Model file for the job. Use its own axes, mm. A direction names the side the tool comes from. Round coordinates to 2 decimals unless told otherwise and drop trailing zeros. Order: outer loops, then holes, each group sorted by start corner. A loop starts at its lowest first (then second) coordinate and runs counter-clockwise, first axis right, second up. Notation, with made-up numbers: M 62.25,80 L 112.25,80 A28 cw 112.25,117 Z; hole C 13,56 d4. An arc over 180 degrees is marked long. Return JSON: item names as keys, results as strings. Group by question number.
Item 1: Pull direction Z, two halves, no side cores. Call faces 1 (the face through (11.745, -3.54, -1.565)), 2 (the face through (0, 2.674, 2)), 3 (the face through (3, 1, 6.975)): pulls with the +Z half, pulls with the -Z half, needs draft (parallel to the pull), parting line crosses it, or undercut.
Item 2: Slice it at D-D on x = 0. Write the cut outline in (y, z) (3 decimals), then the cut area to 3 significant figures.
Item 3: Probe line 1 along Z through (x, y) = (8.25, 1.25) (3 decimals); line 2 along Y through (x, z) = (0, -0.5) (3 decimals); line 3 along Y through (x, z) = (0, 2.75). List the from-to ranges inside material, lowest first.
Item 4: Slice it at A-A on x = 9. Write the cut outline in (y, z) (3 decimals).
Item 5: Slice it at B-B on y = 0. Write the cut outline in (x, z) (1 decimal), then the cut area to 3 significant figures.
Item 6: Pin check, flat tips, straight feed: pin 1 Ø1.1 at (x, z) = (0.5, 1.5) entering from -Y; pin 2 Ø1.1 at (y, z) = (0, 1.5) entering from -X; pin 3 Ø1.9 at (x, z) = (-1, 2.5) entering from +Y. Stop position of each tip, or through.
Item 7: Slice it at C-C on z = -1. Write the cut outline in (x, y) (3 decimals).
Item 8: Which spindle directions (+Z, -Z, +X, -X, +Y, -Y) get a long thin tool onto all of the face, cutting with end or side? Do faces 4 (the face through (0, -2.674, 2)), 5 (the face through (-5.398, 0, 2)), 6 (the face through (-11.795, -3.49, -1.565)). Say none if no direction does.
from build123d import *

# Parameters (mm, degrees)
F0_R      = 1.5
F1_DEPTH  = 3.8
F1_FACE_R = 1.5
F2_DEPTH  = 3.175
F3_R      = 1.5
F4_DEPTH  = 3.175
F5_R      = 1.27
F6_R      = 1.27


with BuildPart() as f1:
    # F0 (on Top) → F1 (new body)
    with BuildSketch(Plane.XY):
        with BuildLine():
            ThreePointArc((5.3975, 2.0388861202), (5.2115128061, 2.4878989263), (4.7625, 2.6738861202))
            Line((4.7625, 2.6738861202), (-4.7625, 2.6738861202))
            ThreePointArc((-4.7625, 2.6738861202), (-5.2115128061, 2.4878989263), (-5.3975, 2.0388861202))
            Line((-5.3975, 2.0388861202), (-5.3975, -2.0388861202))
            ThreePointArc((-5.3975, -2.0388861202), (-5.2115128061, -2.4878989263), (-4.7625, -2.6738861202))
            Line((-4.7625, -2.6738861202), (4.7625, -2.6738861202))
            ThreePointArc((4.7625, -2.6738861202), (5.2115128061, -2.4878989263), (5.3975, -2.0388861202))
            Line((5.3975, -2.0388861202), (5.3975, 2.0388861202))
        make_face()
        Circle(F0_R, mode=Mode.SUBTRACT)
    extrude(amount=F1_DEPTH)

    # F0 (on Top) + F1_face (on face) → F2 (join)
    with BuildSketch(Plane.XY):
        with BuildLine():
            ThreePointArc((12.7, 1.27), (11.7700640303, 3.5150640303), (9.525, 4.445))
            Line((9.525, 4.445), (-9.525, 4.445))
            ThreePointArc((-9.525, 4.445), (-11.7700640303, 3.5150640303), (-12.7, 1.27))
            Line((-12.7, 1.27), (-12.7, -1.27))
            ThreePointArc((-12.7, -1.27), (-11.7700640303, -3.5150640303), (-9.525, -4.445))
            Line((-9.525, -4.445), (9.525, -4.445))
            ThreePointArc((9.525, -4.445), (11.7700640303, -3.5150640303), (12.7, -1.27))
            Line((12.7, -1.27), (12.7, 1.27))
        make_face()
        with BuildLine():
            Line((-4.7625, 2.6738861202), (4.7625, 2.6738861202))
            ThreePointArc((4.7625, 2.6738861202), (5.2115128061, 2.4878989263), (5.3975, 2.0388861202))
            Line((5.3975, 2.0388861202), (5.3975, -2.0388861202))
            ThreePointArc((5.3975, -2.0388861202), (5.2115128061, -2.4878989263), (4.7625, -2.6738861202))
            Line((4.7625, -2.6738861202), (-4.7625, -2.6738861202))
            ThreePointArc((-4.7625, -2.6738861202), (-5.2115128061, -2.4878989263), (-5.3975, -2.0388861202))
            Line((-5.3975, -2.0388861202), (-5.3975, 2.0388861202))
            ThreePointArc((-5.3975, 2.0388861202), (-5.2115128061, 2.4878989263), (-4.7625, 2.6738861202))
        make_face(mode=Mode.SUBTRACT)
    with BuildSketch(Plane(origin=(0, 0, 0), x_dir=(1, 0, 0), z_dir=(0, 0, -1))):
        with BuildLine():
            ThreePointArc((4.7625, -2.6738861202), (5.2115128061, -2.4878989263), (5.3975, -2.0388861202))
            Line((5.3975, -2.0388861202), (5.3975, 2.0388861202))
            ThreePointArc((5.3975, 2.0388861202), (5.2115128061, 2.4878989263), (4.7625, 2.6738861202))
            Line((4.7625, 2.6738861202), (-4.7625, 2.6738861202))
            ThreePointArc((-4.7625, 2.6738861202), (-5.2115128061, 2.4878989263), (-5.3975, 2.0388861202))
            Line((-5.3975, 2.0388861202), (-5.3975, -2.0388861202))
            ThreePointArc((-5.3975, -2.0388861202), (-5.2115128061, -2.4878989263), (-4.7625, -2.6738861202))
            Line((-4.7625, -2.6738861202), (4.7625, -2.6738861202))
        make_face()
        Circle(F1_FACE_R, mode=Mode.SUBTRACT)
    extrude(amount=-F2_DEPTH, dir=(0, 0, 1))

    # F3 (on face) → F4 (join)
    with BuildSketch(Plane.XY.offset(3.8)):
        with BuildLine():
            ThreePointArc((12.7, 1.27), (11.7700640303, 3.5150640303), (9.525, 4.445))
            Line((9.525, 4.445), (-9.525, 4.445))
            ThreePointArc((-9.525, 4.445), (-11.7700640303, 3.5150640303), (-12.7, 1.27))
            Line((-12.7, 1.27), (-12.7, -1.27))
            ThreePointArc((-12.7, -1.27), (-11.7700640303, -3.5150640303), (-9.525, -4.445))
            Line((-9.525, -4.445), (9.525, -4.445))
            ThreePointArc((9.525, -4.445), (11.7700640303, -3.5150640303), (12.7, -1.27))
            Line((12.7, -1.27), (12.7, 1.27))
        make_face()
        with BuildLine():
            ThreePointArc((4.7625, 2.6738861202), (5.2115128061, 2.4878989263), (5.3975, 2.0388861202))
            Line((5.3975, 2.0388861202), (5.3975, -2.0388861202))
            ThreePointArc((5.3975, -2.0388861202), (5.2115128061, -2.4878989263), (4.7625, -2.6738861202))
            Line((4.7625, -2.6738861202), (-4.7625, -2.6738861202))
            ThreePointArc((-4.7625, -2.6738861202), (-5.2115128061, -2.4878989263), (-5.3975, -2.0388861202))
            Line((-5.3975, -2.0388861202), (-5.3975, 2.0388861202))
            ThreePointArc((-5.3975, 2.0388861202), (-5.2115128061, 2.4878989263), (-4.7625, 2.6738861202))
            Line((-4.7625, 2.6738861202), (4.7625, 2.6738861202))
        make_face(mode=Mode.SUBTRACT)
        with BuildLine():
            Line((5.3975, -2.0388861202), (5.3975, 2.0388861202))
            ThreePointArc((5.3975, 2.0388861202), (5.2115128061, 2.4878989263), (4.7625, 2.6738861202))
            Line((4.7625, 2.6738861202), (-4.7625, 2.6738861202))
            ThreePointArc((-4.7625, 2.6738861202), (-5.2115128061, 2.4878989263), (-5.3975, 2.0388861202))
            Line((-5.3975, 2.0388861202), (-5.3975, -2.0388861202))
            ThreePointArc((-5.3975, -2.0388861202), (-5.2115128061, -2.4878989263), (-4.7625, -2.6738861202))
            Line((-4.7625, -2.6738861202), (4.7625, -2.6738861202))
            ThreePointArc((4.7625, -2.6738861202), (5.2115128061, -2.4878989263), (5.3975, -2.0388861202))
        make_face()
        Circle(F3_R, mode=Mode.SUBTRACT)
    extrude(amount=F4_DEPTH)

    # F5
    f5_edges = [f1.edges().sort_by_distance(p)[0] for p in [
        (-1.5, 0, 6.975),
    ]]
    fillet(f5_edges, radius=F5_R)

    # F6
    f6_edges = [f1.edges().sort_by_distance(p)[0] for p in [
        (-1.5, 0, -3.175),
    ]]
    fillet(f6_edges, radius=F6_R)


solid = f1.part
Output values:
{
 "1": {"face 1": "needs draft", "face 2": "undercut", "face 3": "pulls with the +Z half"},
 "2": {"outline": "M -4.445,-3.175 L -2.77,-3.175 A1.27 ccw -1.5,-1.905 L -1.5,5.705 A1.27 ccw -2.77,6.975 L -4.445,6.975 L -4.445,3.8 L -2.674,3.8 L -2.674,0 L -4.445,0 Z; M 1.5,-1.905 A1.27 ccw 2.77,-3.175 L 4.445,-3.175 L 4.445,0 L 2.674,0 L 2.674,3.8 L 4.445,3.8 L 4.445,6.975 L 2.77,6.975 A1.27 ccw 1.5,5.705 Z", "area": "44.9 mm²"},
 "3": {"line 1": "-3.175 to 0, 3.8 to 6.975", "line 2": "-4.445 to -1.5, 1.5 to 4.445", "line 3": "-2.67 to -1.5, 1.5 to 2.67"},
 "4": {"outline": "M -4.445,-3.175 L 4.445,-3.175 L 4.445,0 L -4.445,0 Z; M -4.445,3.8 L 4.445,3.8 L 4.445,6.975 L -4.445,6.975 Z"},
 "5": {"outline": "M -12.7,-3.2 L -2.8,-3.2 A1.3 ccw -1.5,-1.9 L -1.5,5.7 A1.3 ccw -2.8,7 L -12.7,7 L -12.7,3.8 L -5.4,3.8 L -5.4,0 L -12.7,0 Z; M 1.5,-1.9 A1.3 ccw 2.8,-3.2 L 12.7,-3.2 L 12.7,0 L 5.4,0 L 5.4,3.8 L 12.7,3.8 L 12.7,7 L 2.8,7 A1.3 ccw 1.5,5.7 Z", "area": "170 mm²"},
 "6": {"pin 1": "y = -2.67", "pin 2": "x = -5.4", "pin 3": "y = 2.67"},
 "7": {"outline": "M -12.7,-1.27 A3.175 ccw -9.525,-4.445 L 9.525,-4.445 A3.175 ccw 12.7,-1.27 L 12.7,1.27 A3.175 ccw 9.525,4.445 L -9.525,4.445 A3.175 ccw -12.7,1.27 Z; hole C 0,0 d3"},
 "8": {"face 4": "+X, -X, -Y", "face 5": "-X, +Y, -Y", "face 6": "+Z, -Z, -X, -Y"}
}
